Can you work these out from the drawing? Everything is in mm from the part's minimum corner. A direction names the side the tool comes from. Give positions to 0.01 mm unless a question says otherwise; leave off trailing zeros. Loops run counter-clockwise (first coordinate to the right, second up) from the corner with the lowest first, then second, coordinate; pieces in that order, holes last.
Q1. If we section it at B-B (y = 100.5): Please give me the cut outline in (x, z) (1 decimal), plus the area to 3 significant figures.
Q2. For the marked faces 1, 2 and 3, which set-ups out of +Z, -Z, +X, -X, +Y, -Y let a thin tool reach every point of the face, with its end or its side?
Q3. Will these pins go through, and if not, where does the flat tip stop? P1, Ø20.5, axis at x = 83.5, z = 17.5, coming from the +Y side (1 decimal); P2, Ø4, axis at x = 71, z = 114.5, coming from the +Y side; P3, Ø1.5, axis at x = 82.5, z = 91, coming from the +Y side.
Q4. I need wall thicknesses on line 1 (X direction, y = 96.5, z = 53); line 2 (X direction, y = 107, z = 102); line 3 (Z direction, x = 34, y = 67). Which ranges of each line are inside material? Lowest first, please.
Q5. If we section it at A-A (x = 59): Please give me the cut outline in (y, z) (1 decimal), plus the area to 3 significant figures.
Q6. If we section it at C-C (z = 52): Please give me the cut outline in (x, y) (1 decimal), plus the area to 3 significant figures.
Q7. If we section it at D-D (y = 72): Please give me the cut outline in (x, z), plus the area to 3 significant figures.
Q8. We'd pull the mould along Z, two halves only. Please class the marked faces 4, 5 and 6: +Z half, -Z half, draft (parallel to the pull), parting line (faces both ways), or undercut.
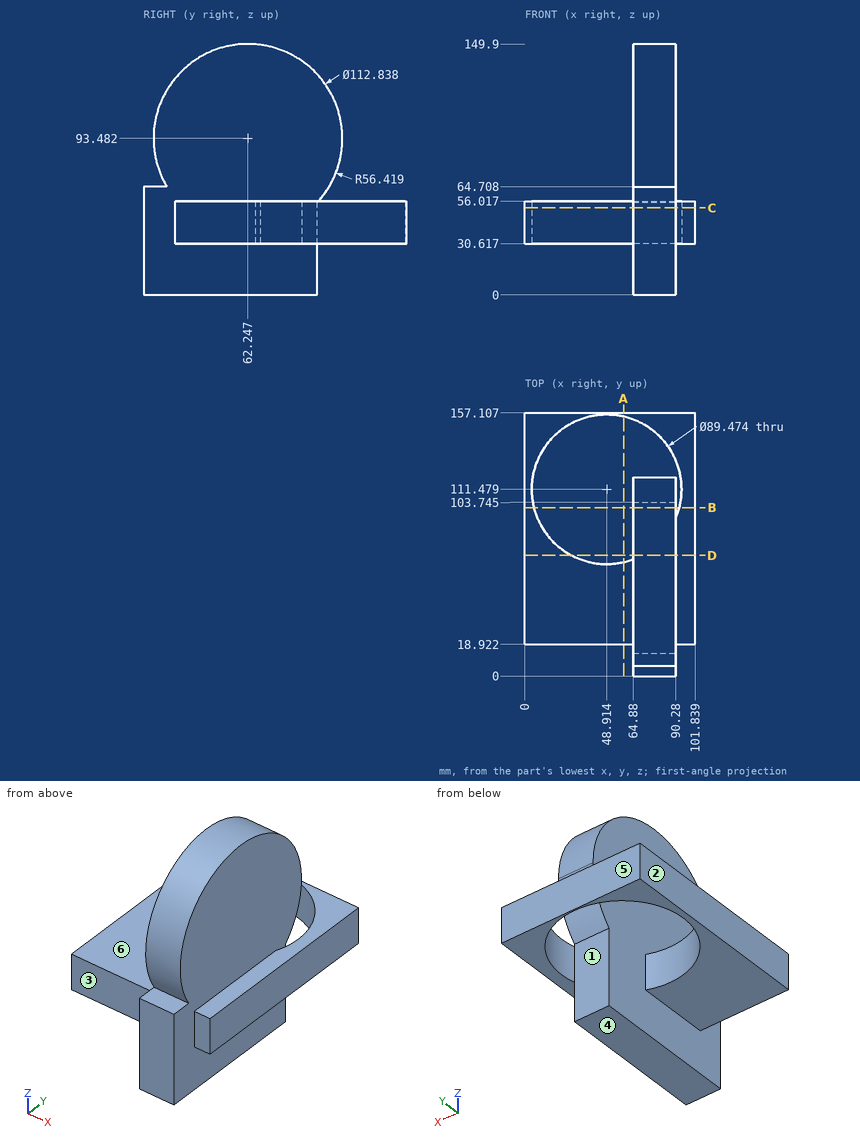
Check sheet entries:
1. outline: (0, 30.6) - (5.5, 30.6) - (5.5, 56) - (0, 56) - close; (64.9, 0) - (90.3, 0) - (90.3, 135) - (64.9, 135) - close; (92.3, 30.6) - (101.8, 30.6) - (101.8, 56) - (92.3, 56) - close
1. area: 3,810 mm2
2. face 1: -Z
2. face 2: +Z, -Z, -X, +Y, -Y
2. face 3: +Z, -Z, -X, -Y
3. P1: stops at y = 103.7
3. P2: stops at y = 115.36
3. P3: stops at y = 118.64
4. line 1: x = 0 to 6.76, 64.88 to 90.28, 91.07 to 101.84
4. line 2: x = 64.88 to 90.28
4. line 3: z = 30.62 to 56.02
5. outline: (18.9, 30.6) - (67.9, 30.6) - (67.9, 56) - (18.9, 56) - close; (155.1, 30.6) - (157.1, 30.6) - (157.1, 56) - (155.1, 56) - close
5. area: 1,300 mm2
6. outline: (0, 18.9) - (64.9, 18.9) - (64.9, 0) - (90.3, 0) - (90.3, 18.9) - (101.8, 18.9) - (101.8, 157.1) - (0, 157.1) - close; hole (64.9, 69.7) - (64.9, 103.7) - (90.3, 103.7) - (90.3, 94.4) arc R44.7 ccw (long way) to start
6. area: 8,900 mm2
7. outline: (0, 30.62) - (27.87, 30.62) - (27.87, 56.02) - (0, 56.02) - close; (64.88, 0) - (90.28, 0) - (90.28, 30.62) - (101.84, 30.62) - (101.84, 56.02) - (90.28, 56.02) - (90.28, 149.05) - (64.88, 149.05) - close
7. area: 4,790 mm2
8. face 4: -Z half
8. face 5: draft
8. face 6: +Z half
